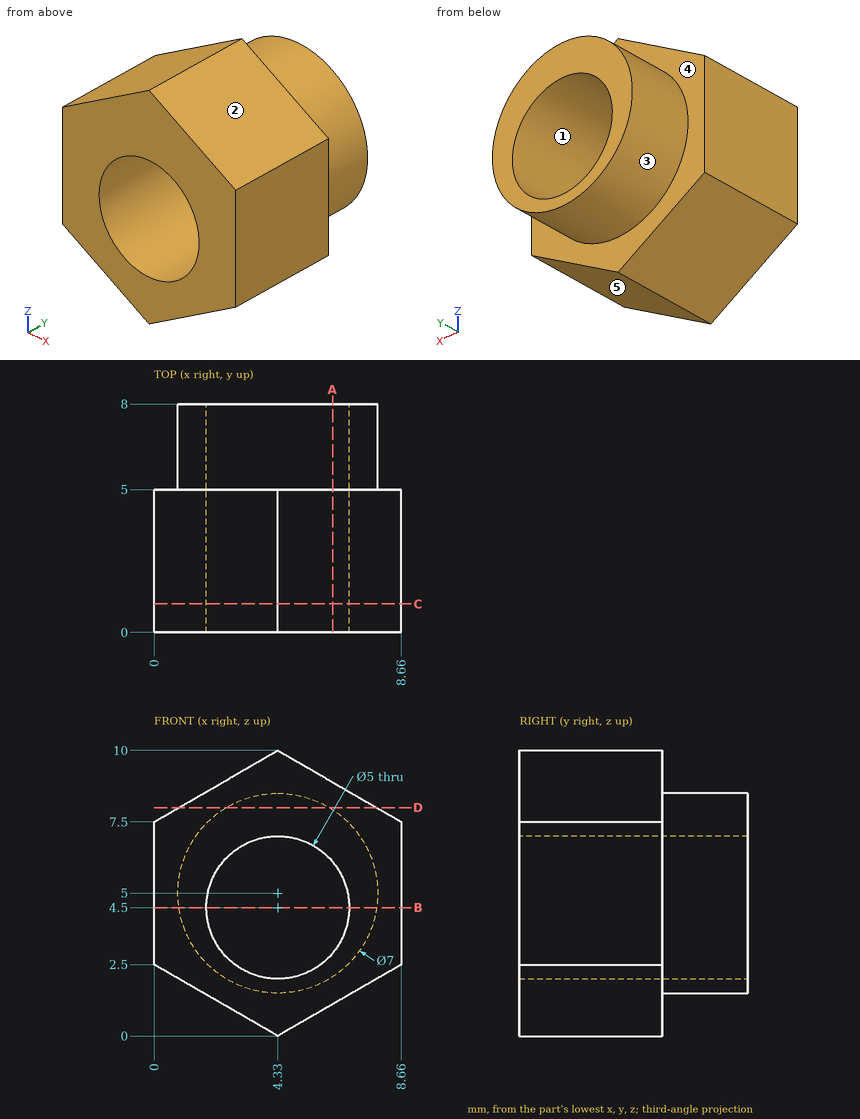
Study the drawing (mm; zero at the part's minimum x, y, z) and answer. A direction names the side the tool comes from. Coordinates: 2 decimals unless noted, no trailing zeros. Write each loop counter-clockwise with the first axis right and the second up, starting at its lowest first coordinate (ties: lowest second). Pieces come first, ordered by that corner, then holes.
Q1. Which of the six approach directions +Z, -Z, +X, -X, +Y, -Y give full straight-line access (tool end or side, diameter ignored) to the marked faces 4 and 5?
Returned:
face 4: +Y
face 5: -Z, +X, +Y, -Y
Q2. Section A-A, the plane x = 6.25 is taken. Write down the section's boundary in (y, z).
Returned:
outline: (0, 1.11) - (5, 1.11) - (5, 2.07) - (8, 2.07) - (8, 2.9) - (0, 2.9) - close; (0, 6.1) - (8, 6.1) - (8, 7.93) - (5, 7.93) - (5, 8.89) - (0, 8.89) - close
Q3. Section C-C, the plane y = 1 is taken. Write down the section's boundary in (x, z).
Returned:
outline: (0, 2.5) - (4.33, 0) - (8.66, 2.5) - (8.66, 7.5) - (4.33, 10) - (0, 7.5) - close; hole circle Ø5 at (4.33, 4.5)
Q4. The mould has two halves that part along X. Classify the marked faces 1, 2 and 3: released by +X, released by -X, zero draft, split by the parting line, or undercut.
Returned:
face 1: undercut
face 2: released by +X
face 3: split by the parting line
Q5. Given P1, Ø3, axis at x = 6, y = 4, coming from the -Z side; P2, Ø2, axis at x = 2, y = 1.5, coming from the -Z side, each flat-ended and moving along its own axis, determine where each tip first touches the part or whether it passes through.
Returned:
P1: stops at z = 0.1
P2: stops at z = 0.77
Q6. Section B-B, the plane z = 4.5 is taken. Write down the section's boundary in (x, y), then the cut area to 3 significant figures.
Returned:
outline: (0, 0) - (1.83, 0) - (1.83, 8) - (0.87, 8) - (0.87, 5) - (0, 5) - close; (6.83, 0) - (8.66, 0) - (8.66, 5) - (7.79, 5) - (7.79, 8) - (6.83, 8) - close
area: 24.1 mm2
Q7. Find the intervals of material crossed by line 1 along X through (y, z) = (4.25, 4.5); line 2 along Y through (x, z) = (0.5, 3.5); line 3 along X through (y, z) = (2.5, 5.5), in increasing order.
Returned:
line 1: x = 0 to 1.83, 6.83 to 8.66
line 2: y = 0 to 5
line 3: x = 0 to 2.04, 6.62 to 8.66
Q8. Section D-D, the plane z = 8 is taken. Write down the section's boundary in (x, y).
Returned:
outline: (0.87, 0) - (7.79, 0) - (7.79, 5) - (6.13, 5) - (6.13, 8) - (2.53, 8) - (2.53, 5) - (0.87, 5) - close
